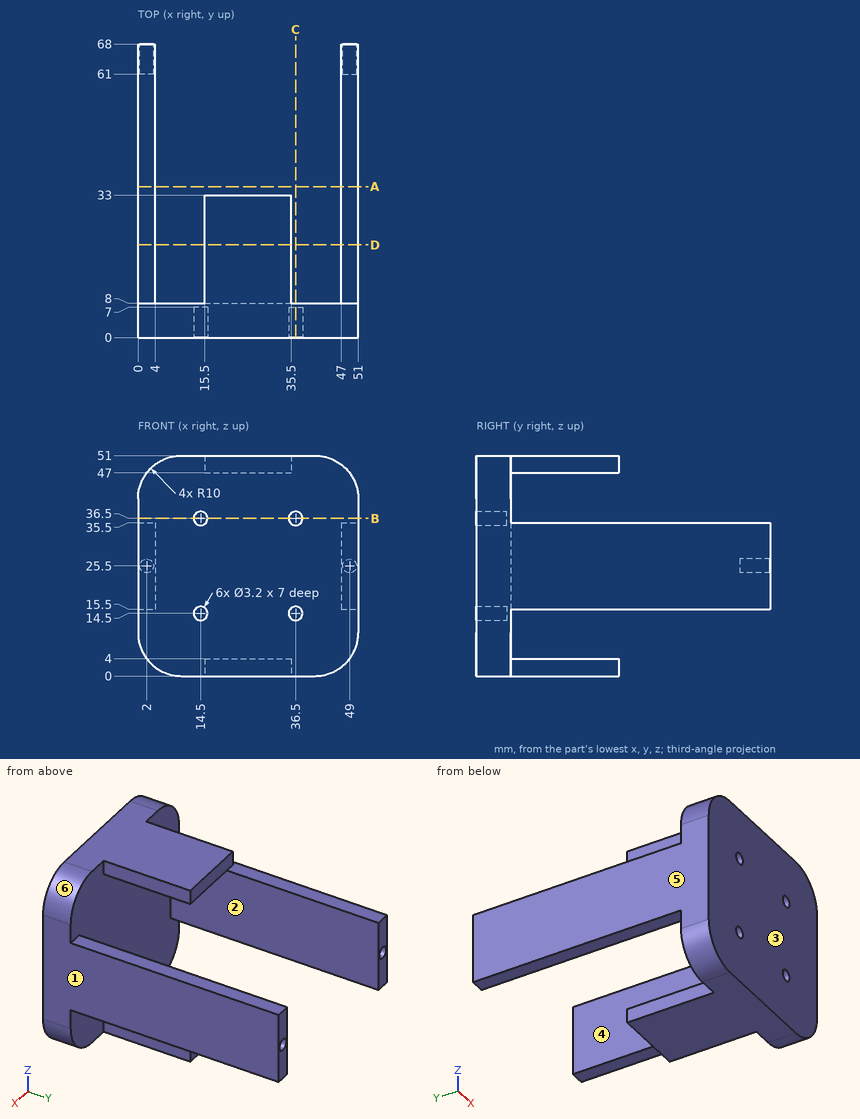
Geometry: see drawing. Coordinates: mm, zero at the bounding-box minimum. A direction names the side the tool comes from. Round coordinates to 2 decimals unless told otherwise and drop trailing zeros. Loops run counter-clockwise (first coordinate to the right, second up) from the corner with the lowest first, then second, coordinate; pieces in that order, holes last. Notation, with made-up numbers: (22, 22) - (65, 22) arc R29 cw to (65, 61) - close; hole circle Ø7 at (-12.75, 50). An arc over 180 degrees is marked (long way). One line per item, written item: value. Start each with the question number.
(1) Section D-D, the plane y = 21.5. Return loops of the section in (x, z).
(2) Contact query for flat-ended pins moving along their axis: P1, Ø2, axis at x = 1.5, y = 30.5, coming from the +Z side; P2, Ø1, axis at x = 39.5, z = 11.5, coming from the +Y side; P3, Ø1, axis at x = 14, z = 36, coming from the -Y side. Output: stop coordinate, or through.
(3) Ray query, line 1 (X direction, y = 64, z = 25.5); line 2 (X direction, y = 4.25, z = 14.5); line 3 (X direction, y = 3, z = 36). Return the intervals inside material, ascending. Write a range as [from, to].
(4) Section B-B, the plane z = 36.5. Return loops of the section in (x, y), plus the area to 3 significant figures.
(5) Section C-C, the plane x = 36.5. Return loops of the section in (y, z), plus the area to 3 significant figures.
(6) Access query for the marked faces 1 and 2. Directions: +Z, -Z, +X, -X, +Y, -Y. A direction counts if a zero-diameter tool reaches every point of the face in a straight line with its end or side. Return the directions, or none.
(7) Section A-A, the plane y = 35. Return loops of the section in (x, z).
(8) Draft query along X for the marked faces 3, 4, 5 and 6. Return one class per face: +X half, -X half, draft (parallel to the pull), parting line (faces both ways), or undercut.
Results below:
1. outline: (0, 15.5) - (4, 15.5) - (4, 35.5) - (0, 35.5) - close; (15.5, 0) - (35.5, 0) - (35.5, 4) - (15.5, 4) - close; (15.5, 47) - (35.5, 47) - (35.5, 51) - (15.5, 51) - close; (47, 15.5) - (51, 15.5) - (51, 35.5) - (47, 35.5) - close
2. P1: z = 35.5
2. P2: y = 8
2. P3: y = 7
3. line 1: [0, 0.4], [3.6, 4], [47, 47.4], [50.6, 51]
3. line 2: [0, 12.9], [16.1, 34.9], [38.1, 51]
3. line 3: [0, 12.98], [16.02, 34.98], [38.02, 51]
4. outline: (0, 0) - (12.9, 0) - (12.9, 7) - (16.1, 7) - (16.1, 0) - (34.9, 0) - (34.9, 7) - (38.1, 7) - (38.1, 0) - (51, 0) - (51, 8) - (0, 8) - close
4. area: 363 mm^2
5. outline: (0, 0) - (8, 0) - (8, 51) - (0, 51) - (0, 38.1) - (7, 38.1) - (7, 34.9) - (0, 34.9) - (0, 16.1) - (7, 16.1) - (7, 12.9) - (0, 12.9) - close
5. area: 363 mm^2
6. face 1: +Z, -Z, +X, +Y, -Y
6. face 2: +Z, -Z, +Y
7. outline: (0, 15.5) - (4, 15.5) - (4, 35.5) - (0, 35.5) - close; (47, 15.5) - (51, 15.5) - (51, 35.5) - (47, 35.5) - close
8. face 3: draft
8. face 4: undercut
8. face 5: -X half
8. face 6: +X half
